from build123d import *

# Parameters (mm, degrees)
FILLET1_R    = 1.5
SKETCH3_W    = 1.42
SKETCH3_H    = 6.6
SKETCH4_W    = 1.42
SKETCH4_H    = 3.15978748
RECPAT_COUNT = 2
RECPAT_ANGLE = 90


with BuildPart() as part:
    # BodySke → Base-Revolve (revolve)
    with BuildSketch(Plane.XY):
        Polygon((0, 0), (0, 5.65), (0.65, 5.65), (3.3, 3), (8, 3), (8, 0), align=None)
    revolve(axis=Axis((-6.35, 0, 0), (1, 0, 0)))

    # Fillet1
    fillet1_edges = [part.edges().sort_by_distance(p)[0] for p in [
        (3.3, -3, 0),
    ]]
    fillet(fillet1_edges, radius=FILLET1_R)

    # Sketch3 → Recess section 0
    with BuildSketch(Plane.ZY):
        Rectangle(SKETCH3_W, SKETCH3_H)
    # Sketch4 → Recess section 1
    with BuildSketch(Plane.ZY.offset(-3.45)):
        Rectangle(SKETCH4_W, SKETCH4_H)
    recess = loft(mode=Mode.SUBTRACT)

    # RecPat: Recess ×2 about axis
    recpat_axis = Axis((0, 0, 0), (1, 0, 0))
    for i in range(1, RECPAT_COUNT):
        add(recess.rotate(recpat_axis, i * RECPAT_ANGLE / (RECPAT_COUNT - 1)), mode=Mode.SUBTRACT)

    # RecCorSke → RecessCore (revolve, cut)
    with BuildSketch(Plane.XY):
        Polygon((0, 0), (0, 1.521747501), (3.45, 1.2805), (3.866059671, 0), align=None)
    revolve(axis=Axis((-3.175, 0, 0), (1, 0, 0)), mode=Mode.SUBTRACT)


solid = part.part
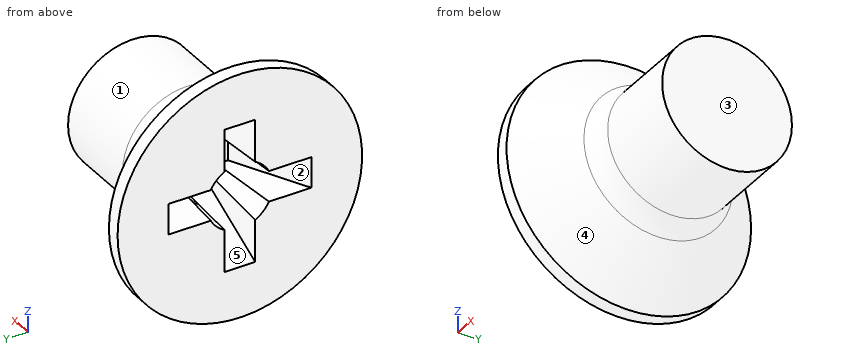
Verification items for the finished model (mm, model axes). Face numbers are marked on the shaded views. A direction names the side the tool comes from. Coordinates: 2 decimals unless noted, no trailing zeros. Write each loop counter-clockwise with the first axis right and the second up, starting at its lowest first coordinate (ties: lowest second). Pieces come first, ordered by that corner, then holes. Notation, with made-up numbers: M 61,52.5 L 75,52.5 A8 ccw 75,67.5 Z; hole C 40,72 d7. An arc over 180 degrees is marked long. Use a Markdown table: item, result.
Q1. Thickness scan on line 1 (X direction, y = 2.5, z = -5); line 2 (Z direction, x = 3, y = -0.75); line 3 (Z direction, x = 1.5, y = 1). Record the ranges inside material, lowest first.
Reply:
| item | result |
|---|---|
| line 1 | x = 0 to 0.71 |
| line 2 | z = -3.23 to -1.08, 1.08 to 3.23 |
| line 3 | z = -4.69 to -1, 1 to 4.69 |
Q2. Draft check along Y on the marked faces 1, 2 and 3. Enter one of: +Y half, -Y half, draft (parallel to the pull), parting line (faces both ways), or undercut.
Reply:
| item | result |
|---|---|
| face 1 | parting line |
| face 2 | undercut |
| face 3 | draft |
Q3. Set-up check for the marked faces 4 and 5: record each of +Z, -Z, +X, -X, +Y, -Y from which the full face is reachable in a straight line by a thin tool's end or side.
Reply:
| item | result |
|---|---|
| face 4 | +X |
| face 5 | -X |
Q4. Sectioned sample at A-A, the plane x = 5.5. Record the boundary of the cut face in (y, z).
Reply:
| item | result |
|---|---|
| outline | C 0,0 d6 |
Q5. Go/stop test with flat-tipped pins: P1, Ø2, axis at x = 2.5, y = 4.5, coming from the +Z side; P2, Ø0.6, axis at y = 0, z = -1.5, coming from the -X side; P3, Ø4, axis at x = 5, z = 0.5, coming from the +Y side; P4, Ø5, axis at y = -0.5, z = 1.5, coming from the -X side. Record where each tip stops, or that it passes through.
Reply:
| item | result |
|---|---|
| P1 | stops at z = 2.44 |
| P2 | stops at x = 3.01 |
| P3 | stops at y = 3.3 |
| P4 | stops at x = 0 |
